For this review, take the finished solid that the model builds, in its own axes (mm). A direction names the side the tool comes from. Give positions to 0.01 mm unless a question says otherwise; leave off trailing zeros. Write each loop counter-clockwise with the first axis right and the second up, starting at its lowest first coordinate (ties: lowest second). Pieces come first, ordered by that corner, then holes. Notation, with made-up numbers: M -10,82 L 41,82 A9 ccw 41,87 Z; hole C 79.5,71.5 d8. An arc over 180 degrees is marked long. Write item = value, one per line.
```python
from build123d import *

# Parameters (mm, degrees)
F0_W     = 457.2
F0_H     = 139.7
F1_DEPTH = 19.05
F2_W     = 19.05
F2_H     = 12.7
F3_DEPTH = 139.701
F4_W     = 19.05
F4_H     = 12.7
F5_DEPTH = 139.701
F7_DEPTH = 19.051


with BuildPart() as f1:
    # F0 (on Front) → F1 (new body)
    with BuildSketch(Plane.XZ):
        with Locations((-228.6, 69.85)):
            Rectangle(F0_W, F0_H)
    extrude(amount=F1_DEPTH)

    # F2 (on face) → F3 (cut, through all)
    with BuildSketch(Plane.XY.offset(139.7)):
        with Locations((-9.525, -6.35)):
            Rectangle(F2_W, F2_H)
    extrude(amount=-F3_DEPTH, mode=Mode.SUBTRACT)

    # F4 (on face) → F5 (cut, through all)
    with BuildSketch(Plane.XY.offset(139.7)):
        with Locations((-447.675, -6.35)):
            Rectangle(F4_W, F4_H)
    extrude(amount=-F5_DEPTH, mode=Mode.SUBTRACT)

    # F6 (on face) → F7 (cut, through all)
    with BuildSketch(Plane.XZ.offset(19.05)):
        with BuildLine():
            Line((-381, 0), (-76.2, 0))
            ThreePointArc((-76.2, 0), (-228.6, 56.515785), (-381, 0))
        make_face()
    extrude(amount=-F7_DEPTH, mode=Mode.SUBTRACT)


solid = f1.part
```
1. We need section A-A, the plane z = 18. Write out the cut boundary in (x, y).
Responses:
outline = M -457.2,-19.05 L -357.14,-19.05 L -357.14,0 L -438.15,0 L -438.15,-12.7 L -457.2,-12.7 Z; M -100.06,-19.05 L 0,-19.05 L 0,-12.7 L -19.05,-12.7 L -19.05,0 L -100.06,0 Z
2. The part is to be moulded in two halves that separate along X. For faces 3 (the face through (-10, -12.7, 71)), 4 (the face through (-19.05, -6, 71)), 5 (the face through (-226.276, -9.658, 56.504)), say which applies: +X half, -X half, draft (parallel to the pull), parting line (faces both ways), or undercut.
Responses:
face_3 = draft
face_4 = +X half
face_5 = undercut
3. For line 1 along Z through (x, y) = (-232.5, -17.25); line 2 along X through (y, z) = (-7.5, 84); line 3 along X through (y, z) = (-2.5, 33.5), list the stretches that pass through material, from the lowest coordinate up. Write a range as from..to.
Responses:
line_1 = 56.48..139.7
line_2 = -438.15..-19.05
line_3 = -438.15..-329.74, -127.46..-19.05
4. We need section B-B, the plane z = 90.5. Write out the cut boundary in (x, y), then the cut area to 3 significant figures.
Responses:
outline = M -457.2,-19.05 L 0,-19.05 L 0,-12.7 L -19.05,-12.7 L -19.05,0 L -438.15,0 L -438.15,-12.7 L -457.2,-12.7 Z
area = 8,230 mm2
5. Machinability: for faces 1 (the face through (-232, -19.05, 86)), 2 (the face through (-438.15, -6, 71)), which of the approach directions +Z, -Z, +X, -X, +Y, -Y give a long, thin tool a straight path to every point of the face, cutting with its end or side? Answer none if there is none.
Responses:
face_1 = +Z, -Z, +X, -X, -Y
face_2 = +Z, -Z, -X, +Y
6. We need section C-C, the plane y = -9.5. Write out the cut boundary in (x, z).
Responses:
outline = M -438.15,0 L -381,0 A233.74 cw -76.2,0 L -19.05,0 L -19.05,139.7 L -438.15,139.7 Z
7. Insertion check: P1, Ø1, axis at x = -99.5, y = -16, coming from the -Z side; P2, Ø4, axis at x = -342, y = -7.5, coming from the -Z side; P3, Ø1, axis at y = -4, z = 120, coming from the +X side. Each pin has a flat end and moves straight along its axis. Give the tip position at first contact, or say it passes through.
Responses:
P1 = 17.3
P2 = 26.04
P3 = -19.05
8. We need section D-D, the plane z = 37.5. Write out the cut boundary in (x, y).
Responses:
outline = M -457.2,-19.05 L -320.95,-19.05 L -320.95,0 L -438.15,0 L -438.15,-12.7 L -457.2,-12.7 Z; M -136.25,-19.05 L 0,-19.05 L 0,-12.7 L -19.05,-12.7 L -19.05,0 L -136.25,0 Z
